from build123d import *

# Parameters (mm, degrees)
SKETCH1_R           = 6.35
SKETCH1_R_2         = 1.8
SKETCH1_W           = 40.171572875
SKETCH1_H           = 16
BOSS_EXTRUDE1_DEPTH = 12.7
FILLET1_R           = 2
CUT_EXTRUDE1_REACH  = 128.18
SKETCH2_R           = 4


with BuildPart() as part:
    # Sketch1 → Boss-Extrude1 (new body)
    with BuildSketch(Plane(origin=(0, 0, 0), x_dir=(1, 0, 0), z_dir=(0, 1, 0))):
        with BuildLine():
            Line((64, 0), (64, 9))
            Line((64, 9), (9, 9))
            ThreePointArc((9, 9), (1.5, 16.5), (9, 24))
            Line((9, 24), (64, 24))
            Line((64, 24), (64, 34))
            Line((64, 34), (-4.907477288, 34))
            ThreePointArc((-4.907477288, 34), (-8.657477288, 35.004809472), (-11.402667816, 37.75))
            Line((-11.402667816, 37.75), (-29.733538863, 69.5))
            ThreePointArc((-29.733538863, 69.5), (-39.857138903, 73.693332437), (-46.527767497, 65))
            Line((-46.527767497, 65), (-46.527767497, -65))
            ThreePointArc((-46.527767497, -65), (-39.857138903, -73.693332437), (-29.733538863, -69.5))
            Line((-29.733538863, -69.5), (3.294228634, -12.294228634))
            ThreePointArc((3.294228634, -12.294228634), (5.705771366, -9.882685902), (9, -9))
            Line((9, -9), (55, -9))
            ThreePointArc((55, -9), (61.363961031, -6.363961031), (64, 0))
        make_face()
        with Locations(Location((0, 0, 0), (0, 0, 270))):
            Circle(SKETCH1_R, mode=Mode.SUBTRACT)
        with Locations(Location((25, 29, 0), (0, 0, 270))):
            Circle(SKETCH1_R_2, mode=Mode.SUBTRACT)
        with Locations(Location((-28.7, 37.9, 0), (0, 0, 270))):
            Circle(SKETCH1_R_2, mode=Mode.SUBTRACT)
        with Locations(Location((-26.1, -47.6, 0), (0, 0, 270))):
            Circle(SKETCH1_R_2, mode=Mode.SUBTRACT)
        with BuildLine():
            Line((52.171572875, 2.828427125), (52.171572875, -2.828427125))
            ThreePointArc((52.171572875, -2.828427125), (59, 0), (52.171572875, 2.828427125))
        make_face(mode=Mode.SUBTRACT)
        with BuildLine():
            Line((-38.563043678, 61.136296695), (-33.664064192, 63.96472382))
            ThreePointArc((-33.664064192, 63.96472382), (-39.527767497, 68.464101615), (-38.563043678, 61.136296695))
        make_face(mode=Mode.SUBTRACT)
        with BuildLine():
            Line((-38.563043678, -61.136296695), (-33.664064192, -63.96472382))
            ThreePointArc((-33.664064192, -63.96472382), (-39.527767497, -68.464101615), (-38.563043678, -61.136296695))
        make_face(mode=Mode.SUBTRACT)
        with Locations((29.085786438, 0)):
            Rectangle(SKETCH1_W, SKETCH1_H, mode=Mode.SUBTRACT)
    extrude(amount=BOSS_EXTRUDE1_DEPTH)

    # Fillet1
    fillet1_edges = [part.edges().sort_by_distance(p)[0] for p in [
        (9, 6.35, -8),
        (9, 6.35, 8),
        (49.171572875, 6.35, 8),
        (49.171572875, 6.35, -8),
    ]]
    fillet(fillet1_edges, radius=FILLET1_R)

    # Sketch2 → Cut-Extrude1 (cut, up to next)
    with BuildSketch(Plane(origin=(0, 0, -34), x_dir=(-1, 0, 0), z_dir=(0, 0, -1)), mode=Mode.PRIVATE) as cut_extrude1_sk1:
        with Locations((-57.65, 6.35)):
            Circle(SKETCH2_R)
    cut_extrude1_tool1 = extrude(cut_extrude1_sk1.sketch, amount=-CUT_EXTRUDE1_REACH, mode=Mode.PRIVATE) & part.part
    add(cut_extrude1_tool1.solids().sort_by_distance((57.65, 6.35, -34))[0], mode=Mode.SUBTRACT)


solid = part.part
Could you check a few things on this model? Use its own coordinates, in mm. A direction names the side the tool comes from. Give positions to 0.01 mm unless a question says otherwise; leave off trailing zeros. Order: outer loops, then holes, each group sorted by start corner. A loop starts at its lowest first (then second) coordinate and runs counter-clockwise, first axis right, second up. Notation, with made-up numbers: (-8, 43) -> (18, 43) arc R24 ccw to (18, 65) -> close; hole circle Ø10 at (85.25, 4). An arc over 180 degrees is marked (long way). Answer in a Markdown table with one row per item. Add a question column.
Item 1: Imagine slicing it at D-D (z = -16.5). List the corners of the cut face in (x, y) for me, and give its area (3 significant figures).
Item 2: Imagine slicing it at B-B (y = 6.35). Count the separate pieces of the cut face and the enclosed holes in it, and give its area (3 significant figures).
Item 3: For faces 4 (the flat face through (-17, 12.7, -17)), 5 (the flat face through (36, 6, -24)), 6 (the flat face through (30, 6, -34)), 7 (the flat face through (52.172, 6, 0)), which set-ups out of +Z, -Z, +X, -X, +Y, -Y let a thin tool reach every point of the face, with its end or its side?
Item 4: Imagine slicing it at C-C (x = -2). List the corners of the cut face in (y, z) for me.
Item 5: Please list where these lines run through material, in increasing order: probe 1 along X at (y, z) = (7, 0); probe 2 along Z at (x, y) = (55, 3); probe 3 along Z at (x, y) = (15, 11.5).
Item 6: Imagine slicing it at A-A (x = 42). List the corners of the cut face in (y, z) for me.
Item 7: We'd pull the mould along Z, two halves only. Please class faces 1 (the flat face through (37, 6, -9)), 2 (the flat face through (64, 6, -29)), 3 (the flat face through (32, 6, 9)): pulls with the +Z half, pulls with the -Z half, needs draft (parallel to the pull), parting line crosses it, or undercut.
Item 8: I'm going to push flat-ended pins straight in: P1, Ø6.5, axis at x = 40, y = 7.5, coming from the -Z side; P2, Ø5, axis at x = 43, y = 3, coming from the +Z side; P3, Ø3, axis at x = -28.7, z = -37.9, coming from the -Y side; P4, Ø3, axis at y = 6.5, z = 30, coming from the +X side. Where does each tip first touch, or does it pass through?
Result:
| question | item | result |
|---|---|---|
| 1 | outline | (-46.53, 0) -> (1.5, 0) -> (1.5, 12.7) -> (-46.53, 12.7) -> close |
| 1 | area | 610 mm2 |
| 2 | separate pieces | 2 |
| 2 | enclosed holes | 8 |
| 2 | area | 5,940 mm2 |
| 3 | face 4 | +Z, -Z, +X, -X, +Y |
| 3 | face 5 | +X, +Y, -Y |
| 3 | face 6 | -Z, +X, +Y, -Y |
| 3 | face 7 | +Y, -Y |
| 4 | outline | (0, -34) -> (12.7, -34) -> (12.7, -6.03) -> (0, -6.03) -> close; (0, 6.03) -> (12.7, 6.03) -> (12.7, 21.46) -> (0, 21.46) -> close |
| 5 | probe 1 | -46.53 to -6.35, 6.35 to 9, 49.17 to 52.17, 59 to 64 |
| 5 | probe 2 | -34 to -24, -9 to -4, 4 to 9 |
| 5 | probe 3 | -34 to -24, -9 to -8, 8 to 9 |
| 6 | outline | (0, -34) -> (12.7, -34) -> (12.7, -24) -> (0, -24) -> close; (0, -9) -> (12.7, -9) -> (12.7, -8) -> (0, -8) -> close; (0, 8) -> (12.7, 8) -> (12.7, 9) -> (0, 9) -> close |
| 7 | face 1 | undercut |
| 7 | face 2 | needs draft |
| 7 | face 3 | pulls with the +Z half |
| 8 | P1 | z = -34 |
| 8 | P2 | z = 9 |
| 8 | P3 | through |
| 8 | P4 | x = -6.06 |
